Can you work these out from the model? Positions are in its coordinate system, mm. Face numbers are marked on the shaded views. A direction names the side the tool comes from. Give positions to 0.01 mm unless a question says otherwise; leave off trailing zeros. Write each loop counter-clockwise with the first axis right and the second up, starting at its lowest first coordinate (ties: lowest second). Pieces come first, ordered by that corner, then holes.
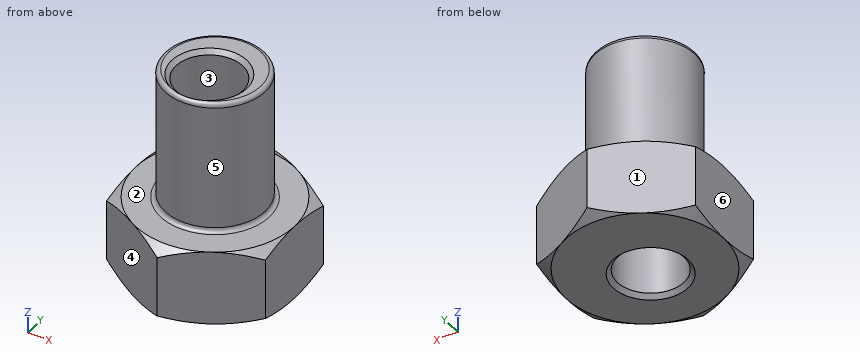
from build123d import *

# Parameters (mm, degrees)
HEX_EXTRUDE_DEPTH        = 9
SKETCH4_OUTSIDE_W        = 132.26
SKETCH4_OUTSIDE_H        = 135.2
SKETCH4_OUTSIDE_R        = 9.5
HEX_CUT1_DEPTH           = 29.906458333
HEX_CUT1_DRAFT           = -60
SKETCH5_OUTSIDE_W        = 106.952
SKETCH5_OUTSIDE_H        = 109.892
SKETCH5_OUTSIDE_R        = 9.5
HEX_CUT2_DEPTH           = 22.600540117
HEX_CUT2_DRAFT           = -60
SKETCH6_R                = 4
ECCENTRIC_HOLE_CUT_DEPTH = 29.906458333
FILLET_2_R               = 0.508
CHAMFER_2_SIZE           = 0.5


with BuildPart() as part:
    # Sketch2 → Body Revolve (revolve)
    with BuildSketch(Plane(origin=(0, 0, 0), x_dir=(0, 0, -1), z_dir=(1, 0, 0)), mode=Mode.PRIVATE) as body_revolve_sk:
        Polygon((-12.5, 0), (12.5, 0), (12.5, 9.5), (3.5, 9.5), (3.5, 6), (-12.5, 6), align=None)
    revolve(body_revolve_sk.sketch.rotate(Axis((0, 0, 12.5), (0, 0, -1)), 90), axis=Axis((0, 0, 12.5), (0, 0, -1)))

    # Sketch3 → Hex Extrude (add)
    with BuildSketch(Plane(origin=(0, 0, -12.5), x_dir=(-1, 0, 0), z_dir=(0, 0, -1))):
        Polygon((0, 10.969655115), (-9.5, 5.484827557), (-9.5, -5.484827557), (0, -10.969655115), (9.5, -5.484827557), (9.5, 5.484827557), align=None)
    extrude(amount=-HEX_EXTRUDE_DEPTH)


with BuildPart() as hex_cut1_tool:
    # Sketch4 outside → Hex Cut1 (with draft: the straight prism first)
    with BuildSketch(Plane(origin=(0, 0, -12.5), x_dir=(-1, 0, 0), z_dir=(0, 0, -1))):
        Rectangle(SKETCH4_OUTSIDE_W, SKETCH4_OUTSIDE_H)
        Circle(SKETCH4_OUTSIDE_R, mode=Mode.SUBTRACT)
    extrude(amount=-HEX_CUT1_DEPTH)
    # Hex Cut1: the draft: its side faces are tilted about the plane it starts from
    hex_cut1_sides = [hex_cut1_tool.faces().sort_by_distance(p)[0] for p in [
        (0, -67.6, 2.453229166),
        (-66.13, 0, 2.453229166),
        (0, 67.6, 2.453229166),
        (66.13, 0, 2.453229166),
        (9.5, 0, 2.453229166),
    ]]
    draft(hex_cut1_sides, Plane(origin=(0, 0, -12.5), x_dir=(-1, 0, 0), z_dir=(0, 0, -1)), HEX_CUT1_DRAFT)


with BuildPart() as part_1:
    add(part.part)

    # Hex Cut1: cut by hex_cut1_tool
    add(hex_cut1_tool.part, mode=Mode.SUBTRACT)


with BuildPart() as hex_cut2_tool:
    # Sketch5 outside → Hex Cut2 (with draft: the straight prism first)
    with BuildSketch(Plane.XY.offset(-3.5)):
        Rectangle(SKETCH5_OUTSIDE_W, SKETCH5_OUTSIDE_H)
        Circle(SKETCH5_OUTSIDE_R, mode=Mode.SUBTRACT)
    extrude(amount=-HEX_CUT2_DEPTH)
    # Hex Cut2: the draft: its side faces are tilted about the plane it starts from
    hex_cut2_sides = [hex_cut2_tool.faces().sort_by_distance(p)[0] for p in [
        (0, -54.946, -14.800270058),
        (53.476, 0, -14.800270058),
        (0, 54.946, -14.800270058),
        (-53.476, 0, -14.800270058),
        (-9.5, 0, -14.800270058),
    ]]
    draft(hex_cut2_sides, Plane.XY.offset(-3.5), HEX_CUT2_DRAFT)


with BuildPart() as part_2:
    add(part_1.part)

    # Hex Cut2: cut by hex_cut2_tool
    add(hex_cut2_tool.part, mode=Mode.SUBTRACT)

    # Sketch6 → Eccentric Hole Cut (cut, through all)
    with BuildSketch(Plane.XY.offset(12.5)):
        with Locations((0, -1.07)):
            Circle(SKETCH6_R)
    extrude(amount=-ECCENTRIC_HOLE_CUT_DEPTH, mode=Mode.SUBTRACT)

    # Fillet 2
    fillet_2_edges = [part_2.edges().sort_by_distance(p)[0] for p in [
        (-6, 0, 12.5),
        (-6, 0, -3.5),
    ]]
    fillet(fillet_2_edges, radius=FILLET_2_R)

    # Chamfer 2
    # the kernel refuses this chamfer: 0.5 mm, written as the material it takes off along each edge
    with BuildSketch(Plane(origin=(0, -1.07, -12.5), x_dir=(1, 0, 0), z_dir=(0, -1, 0))) as chamfer_2_piece_1:
        Polygon((4, CHAMFER_2_SIZE), (4 + CHAMFER_2_SIZE, 0), (4, 0), align=None)
    revolve(axis=Axis((0, -1.07, -12.5), (0, 0, 1)), mode=Mode.SUBTRACT)
    with BuildSketch(Plane(origin=(0, -1.07, 12.5), x_dir=(1, 0, 0), z_dir=(0, -1, 0))) as chamfer_2_piece_2:
        Polygon((4 + CHAMFER_2_SIZE, 0), (4, -CHAMFER_2_SIZE), (4, 0), align=None)
    revolve(axis=Axis((0, -1.07, 12.5), (0, 0, 1)), mode=Mode.SUBTRACT)


solid = part_2.part
(1) For the marked faces 5 and 6, which set-ups out of +Z, -Z, +X, -X, +Y, -Y let a thin tool reach every point of the face, with its end or its side?
Returned:
face 5: +Z
face 6: +Z, -Z, -X, +Y, -Y
(2) Will these pins go through, and if not, where does the flat tip stop? P1, Ø3, axis at x = 4.5, z = 0.5, coming from the -Y side; P2, Ø1.5, axis at x = 5, z = -5.5, coming from the -Y side; P3, Ø1.5, axis at y = 8.5, z = -3.5, coming from the -X side; P4, Ø1, axis at y = 8, z = 4.5, coming from the -X side.
Returned:
P1: stops at y = -5.2
P2: stops at y = -8.52
P3: stops at x = -5.58
P4: passes through
(3) Imagine slicing it at A-A, the plane z = -5. Write out the boundary of the cut face in (x, y).
Returned:
outline: (-9.5, -5.48) - (0, -10.97) - (9.5, -5.48) - (9.5, 5.48) - (0, 10.97) - (-9.5, 5.48) - close; hole circle Ø8 at (0, -1.07)
(4) If I drill on L1, parallel to Y at x = 0, z = 2; L2, parallel to Z at x = 0.75, y = -7.25; L3, parallel to Y at x = 2.5, z = -9.5, over which ranges is the centre line in solid material (lowest first)?
Returned:
L1: y = -6 to -5.07, 2.93 to 6
L2: z = -12.5 to -3.5
L3: y = -9.53 to -4.19, 2.05 to 9.53
(5) If we mould it in two halves opening along Y, with no side actions, what happens to the marked faces 1, 2, 3 and 4? For each: +Y half, -Y half, draft (parallel to the pull), parting line (faces both ways), or undercut.
Returned:
face 1: +Y half
face 2: draft
face 3: undercut
face 4: -Y half
(6) Imagine slicing it at B-B, the plane z = -1.75. Write out the boundary of the cut face in (x, y), plus the area to 3 significant figures.
Returned:
outline: circle Ø12 at (0, 0); hole circle Ø8 at (0, -1.07)
area: 62.8 mm2
